from build123d import *

# Parameters (mm, degrees)
F1_DEPTH = 10.2
F2_R     = 6.25
F3_DEPTH = 10.201


with BuildPart() as f1:
    # F0 (on Top) → F1 (new body)
    with BuildSketch(Plane.XY):
        Polygon((15.854947, 15.895053), (-47.645053, 15.895053), (-15.854947, -15.895053), (47.645053, -15.895053), align=None)
    extrude(amount=F1_DEPTH)

    # F2 (on face) → F3 (cut, through all)
    with BuildSketch(Plane.XY.offset(10.2)):
        Circle(F2_R)
    extrude(amount=-F3_DEPTH, mode=Mode.SUBTRACT)


solid = f1.part
Model file for the job. Use its own axes, mm. Give positions to 0.01 mm unless a question says otherwise; leave off trailing zeros. Order: outer loops, then holes, each group sorted by start corner. A loop starts at its lowest first (then second) coordinate and runs counter-clockwise, first axis right, second up. Notation, with made-up numbers: (69.5, -27) - (101.5, -27) arc R25 cw to (101.5, 8) - close; hole circle Ø8 at (-19, -34.75). An arc over 180 degrees is marked (long way). Return JSON: item names as keys, results as strings.
1) Probe line 1 (Y direction, x = 0, z = 6); line 2 (X direction, y = 1.5, z = 0.5); line 3 (X direction, y = -1.5, z = 9.5). List the from-to ranges inside material, lowest first. Write a range as from..to.
Geometry says:
{"line 1": "-15.9..-6.25, 6.25..15.9", "line 2": "-33.25..-6.07, 6.07..30.25", "line 3": "-30.25..-6.07, 6.07..33.25"}
2) Flat gauge pins, fed straight in: P1, Ø11, axis at x = 0, y = 0, coming from the +Z side; P2, Ø5, axis at y = 11.5, z = 7.5, coming from the -X side; P3, Ø2, axis at x = -21.5, z = 8, coming from the -Y side. Where does each tip first touch, or does it go through?
Geometry says:
{"P1": "through", "P2": "x = -45.75", "P3": "y = -11.25"}
3) Cut at B-B, the plane x = 0. Give the cut face in (y, z).
Geometry says:
{"outline": "(-15.9, 0) - (-6.25, 0) - (-6.25, 10.2) - (-15.9, 10.2) - close; (6.25, 0) - (15.9, 0) - (15.9, 10.2) - (6.25, 10.2) - close"}
4) Cut at A-A, the plane y = 0. Give the cut face in (x, z), plus the area to 3 significant figures.
Geometry says:
{"outline": "(-31.75, 0) - (-6.25, 0) - (-6.25, 10.2) - (-31.75, 10.2) - close; (6.25, 0) - (31.75, 0) - (31.75, 10.2) - (6.25, 10.2) - close", "area": "520 mm²"}
5) Pull direction Y, two halves, no side cores. Call faces 1 (the cylindrical face through (5.96, 1.88, 5.17)), 2 (the flat face through (-1, -7, 0)), 3 (the flat face through (-15, 15.895, 5)), 4 (the flat face through (15, -15.895, 5)): pulls with the +Y half, pulls with the -Y half, needs draft (parallel to the pull), parting line crosses it, or undercut.
Geometry says:
{"face 1": "undercut", "face 2": "needs draft", "face 3": "pulls with the +Y half", "face 4": "pulls with the -Y half"}
6) Cut at C-C, the plane z = 8.25. Give the cut face in (x, y).
Geometry says:
{"outline": "(-47.65, 15.9) - (-15.85, -15.9) - (47.65, -15.9) - (15.85, 15.9) - close; hole circle Ø12.5 at (0, 0)"}
